```python
from build123d import *


with BuildPart() as part:
    # Reconstructed nominal axial profile → Native revolved geometry (revolve)
    with BuildSketch(Plane.XY, mode=Mode.PRIVATE) as native_revolved_geometry_sk:
        Polygon((8.6, -78), (8.6, -80.5), (8, -80.5), (8, -278), (10, -278), (10, -82.339745962), (15, -81), (15, -78), align=None)
    revolve(native_revolved_geometry_sk.sketch.rotate(Axis((0, -500, 0), (0, 1, 0)), 90), axis=Axis((0, -500, 0), (0, 1, 0)))


solid = part.part
```
Design review of the part built by this model. Coordinates are the model's own, in mm. A direction names the side the tool comes from. Coordinates: 2 decimals unless noted, no trailing zeros. Write each loop counter-clockwise with the first axis right and the second up, starting at its lowest first coordinate (ties: lowest second). Pieces come first, ordered by that corner, then holes.
1) Machinability: for faces 4 (the cylindrical face through (0, -179, 10)), 5 (the cylindrical face through (-0.38, -79.27, 8.59)), 6 (the flat face through (-8.2, -278, 0)), which of the approach directions +Z, -Z, +X, -X, +Y, -Y give a long, thin tool a straight path to every point of the face, cutting with its end or side? Answer none if there is none.
2) Add section C-C (y = -100.5). Write out the cut boundary in (x, z).
3) To check wall thickness, follow L1, parallel to X at y = -205, z = 0; L2, parallel to X at y = -79.2, z = 0; L3, parallel to Z at x = 5.5, y = -256. State the ranges of each line that lie inside material, in increasing order.
4) Insertion check: pin 1 (4 mm diameter, centred on x = 9.5, z = 9, fed in from -Y); pin 2 (1.5 mm diameter, centred on y = -141, z = 9.5, fed in from +X); pin 3 (10 mm diameter, centred on y = -156, z = 3.5, fed in from +X). Each pin has a flat end and moves straight along its axis. Give the tip position at first contact, or say it passes through.
5) Mouldability with a two-part tool opening along X and no side actions: class faces 1 (the flat face through (6.5, -78, -6.5)), 2 (the conical face through (9.149, -82.256, -4.759)), 3 (the cylindrical face through (7.81, -180.63, 1.73)) as +X half, -X half, draft (parallel to the pull), parting line (faces both ways), or undercut.
6) Add section B-B (x = 0). Write out the cut boundary in (y, z), plus the area to 3 significant figures.
7) Add section A-A (z = 0). Write out the cut boundary in (x, y).
Check result:
1. face 4: -Y
1. face 5: +Y
1. face 6: +Z, -Z, +X, -X, -Y
2. outline: circle Ø20 at (0, 0); hole circle Ø16 at (0, 0)
3. L1: x = -10 to -8, 8 to 10
3. L2: x = -15 to -8.6, 8.6 to 15
3. L3: z = -8.35 to -5.81, 5.81 to 8.35
4. pin 1: stops at y = -82.05
4. pin 2: stops at x = 4.84
4. pin 3: stops at x = 10
5. face 1: draft
5. face 2: parting line
5. face 3: undercut
6. outline: (-278, -10) - (-82.34, -10) - (-81, -15) - (-78, -15) - (-78, -8.6) - (-80.5, -8.6) - (-80.5, -8) - (-278, -8) - close; (-278, 8) - (-80.5, 8) - (-80.5, 8.6) - (-78, 8.6) - (-78, 15) - (-81, 15) - (-82.34, 10) - (-278, 10) - close
6. area: 834 mm2
7. outline: (-15, -81) - (-10, -82.34) - (-10, -278) - (-8, -278) - (-8, -80.5) - (-8.6, -80.5) - (-8.6, -78) - (-15, -78) - close; (8, -278) - (10, -278) - (10, -82.34) - (15, -81) - (15, -78) - (8.6, -78) - (8.6, -80.5) - (8, -80.5) - close
